from build123d import *

# Parameters (mm, degrees)
SKETCH1_R           = 1.5
SKETCH1_W           = 6.4
SKETCH1_H           = 9.8
SKETCH1_W_2         = 9.8
SKETCH1_H_2         = 6.4
BOSS_EXTRUDE1_DEPTH = 6.4


with BuildPart() as part:
    # Sketch1 → Boss-Extrude1 (new body)
    with BuildSketch(Plane(origin=(0, 0, 0), x_dir=(0, 0, -1), z_dir=(1, 0, 0))):
        Polygon((-132.823391234, 28.785955079), (114.976608766, 28.785955079), (151.076608766, -7.314044921), (151.076608766, 204.295266909), (-55.414079404, 204.295266909), (-168.923391234, 90.785955079), (-168.923391234, -7.314044921), align=None)
        with Locations((144.275039161, 57.480587849)):
            Circle(SKETCH1_R, mode=Mode.SUBTRACT)
        with Locations((144.275039161, 157.480587849)):
            Circle(SKETCH1_R, mode=Mode.SUBTRACT)
        with Locations((27.831264681, 197.495266909)):
            Circle(SKETCH1_R, mode=Mode.SUBTRACT)
        with Locations((-79.85274236, 170.239957095)):
            Circle(SKETCH1_R, mode=Mode.SUBTRACT)
        with Locations((-129.350217044, 120.742482412)):
            Circle(SKETCH1_R, mode=Mode.SUBTRACT)
        with Locations((-162.121821629, 57.480587849)):
            Circle(SKETCH1_R, mode=Mode.SUBTRACT)
        with Locations((144.275039161, 142.480587849)):
            Rectangle(SKETCH1_W, SKETCH1_H, mode=Mode.SUBTRACT)
        with Locations((144.275039161, 172.480587849)):
            Rectangle(SKETCH1_W, SKETCH1_H, mode=Mode.SUBTRACT)
        with Locations((144.275039161, 72.480587849)):
            Rectangle(SKETCH1_W, SKETCH1_H, mode=Mode.SUBTRACT)
        with Locations((144.275039161, 42.480587849)):
            Rectangle(SKETCH1_W, SKETCH1_H, mode=Mode.SUBTRACT)
        with Locations((42.831264681, 197.495266909)):
            Rectangle(SKETCH1_W_2, SKETCH1_H_2, mode=Mode.SUBTRACT)
        with Locations((12.831264681, 197.495266909)):
            Rectangle(SKETCH1_W_2, SKETCH1_H_2, mode=Mode.SUBTRACT)
        Polygon((-68.044023742, 186.574153746), (-63.518540343, 182.048670346), (-70.448186798, 175.119023891), (-74.973670198, 179.64450729), align=None, mode=Mode.SUBTRACT)
        Polygon((-96.186873634, 158.431303855), (-89.257227178, 165.36095031), (-84.731743778, 160.835466911), (-91.661390234, 153.905820455), align=None, mode=Mode.SUBTRACT)
        Polygon((-113.016080404, 132.551130285), (-117.541563803, 137.076613685), (-124.471210259, 130.146967229), (-119.945726859, 125.62148383), align=None, mode=Mode.SUBTRACT)
        Polygon((-138.754767239, 115.863410249), (-145.684413695, 108.933763794), (-141.158930295, 104.408280394), (-134.229283839, 111.33792685), align=None, mode=Mode.SUBTRACT)
        with Locations((-162.121821629, 42.480587849)):
            Rectangle(SKETCH1_W, SKETCH1_H, mode=Mode.SUBTRACT)
        with Locations((-162.121821629, 72.480587849)):
            Rectangle(SKETCH1_W, SKETCH1_H, mode=Mode.SUBTRACT)
    extrude(amount=BOSS_EXTRUDE1_DEPTH)


solid = part.part
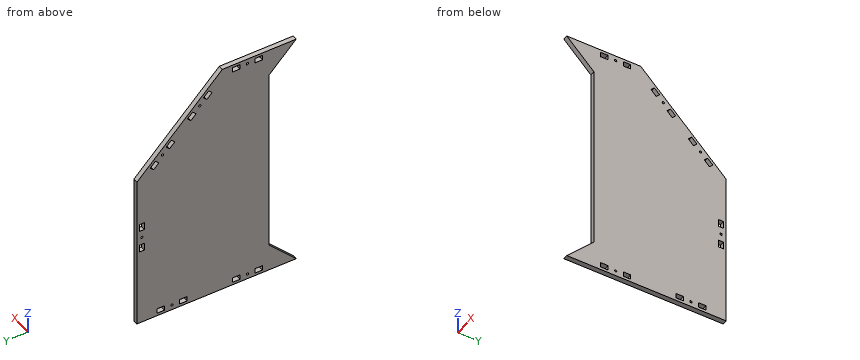
Source: CAD feature listing. Evaluate the final solid. Frame: model axes, mm. Give positions to 0.01 mm unless a question says otherwise; leave off trailing zeros. Loops run counter-clockwise (first coordinate to the right, second up) from the corner with the lowest first, then second, coordinate; pieces in that order, holes last. Notation, with made-up numbers: (77, -37.75) -> (101, -37.75) arc R21 ccw to (101, -32.75) -> close; hole circle Ø1 at (-5.75, 63.5). An arc over 180 degrees is marked (long way). Use a Markdown table: item, result. Add a question column.
1) Section query C-C, the plane x = 3.75. Count the separate pieces of the cut face and the enclosed holes in it, then the cut area to 3 significant figures.
2) Section query D-D, the plane z = 107. Return the cut outline in (x, y), then the cut area to 3 significant figures.
3) Section query B-B, the plane z = 13. Return the cut outline in (x, y), then the cut area to 3 significant figures.
4) Line query: line 1 along Z through (x, y) = (3, 71); line 2 along Y through (x, z) = (1, -68.5); line 3 along Z through (x, y) = (6, 155). Output: solid intervals per line, ascending. Write a range as [from, to].
5) Section query A-A, the plane y = 73. Return the cut outline in (x, z).
6) First-contact query: pin 1 (3 mm diameter, centred on x = 3, z = -5.5, fed in from -Y); pin 2 (1 mm diameter, centred on x = 1.5, y = 181.5, fed in from +Z); pin 3 (3 mm diameter, centred on x = 3.5, y = 171.5, fed in from +Z). Flat tips, straight axial feed; report the tip coordinate or a pass-through.
Numbers:
| question | item | result |
|---|---|---|
| 1 | separate pieces | 1 |
| 1 | enclosed holes | 18 |
| 1 | area | 50,200 mm2 |
| 2 | outline | (0, 28.79) -> (6.4, 28.79) -> (6.4, 152.71) -> (0, 152.71) -> close |
| 2 | area | 793 mm2 |
| 3 | outline | (0, 28.79) -> (6.4, 28.79) -> (6.4, 204.3) -> (0, 204.3) -> close |
| 3 | area | 1,120 mm2 |
| 4 | line 1 | z = [-151.08, -147.48], [-141.08, 158.92], [165.32, 168.92] |
| 4 | line 2 | y = [28.79, 204.3] |
| 4 | line 3 | z = [-151.08, 90.57], [92.76, 104.71] |
| 5 | outline | (0, -151.08) -> (6.4, -151.08) -> (6.4, -147.48) -> (0, -147.48) -> close; (0, -141.08) -> (6.4, -141.08) -> (6.4, 158.92) -> (0, 158.92) -> close; (0, 165.32) -> (6.4, 165.32) -> (6.4, 168.92) -> (0, 168.92) -> close |
| 6 | pin 1 | stops at y = 28.79 |
| 6 | pin 2 | stops at z = 78.71 |
| 6 | pin 3 | stops at z = 89.71 |
